from build123d import *

# Parameters (mm, degrees)
CIRPATTERN1_COUNT        = 8
LPATTERN1_START          = -24.818843944
LPATTERN1_OUTLINE_R      = 41.275
LPATTERN1_OUTLINE_R_2    = 38.453474767
LPATTERN1_DEPTH          = 5.187687888
LPATTERN1_START_2        = -12.118843944
LPATTERN1_2_OUTLINE_R    = 41.275
LPATTERN1_2_OUTLINE_R_2  = 38.453474767
LPATTERN1_2_DEPTH        = 5.187687888
Q_0_332_DIAMETER_HOLE1_D = 8.4328


# Read off the part's stored shape, not the designer's step: LPattern1
with BuildPart() as part:
    # Sketch1 → Revolve1 (revolve)
    with BuildSketch(Plane.XY, mode=Mode.PRIVATE) as revolve1_sk:
        Polygon((-41.275, -40.64), (-41.275, 0), (-34.925, 0), (-34.925, -25.4), (-13.91158, -25.4), (-13.91158, -74.93), (-8.90651, -74.93), (-8.90651, -88.392), (-19.05, -88.392), (-19.05, -40.64), align=None)
    revolve(revolve1_sk.sketch.rotate(Axis((0, 0, 0), (0, 1, 0)), 270), axis=Axis((0, 0, 0), (0, 1, 0)))

    # Sketch8 → 1/4-20 Tapped Hole1 (revolve, cut)
    with BuildSketch(Plane(origin=(38.133127704, -34.29, -15.795258671), x_dir=(-0.38268343236509045, 0, -0.9238795325112865), z_dir=(0, 1, 0))):
        Polygon((0, 0), (0, 20.583816902), (2.5527, 19.05), (2.5527, 0), align=None)
    f_1_4_20_tapped_hole1 = revolve(axis=Axis((43.999762736, -34.29, -18.225298466), (-0.9238795325112865, 0, 0.38268343236509045)), mode=Mode.SUBTRACT)

    # CirPattern1: 1/4-20 Tapped Hole1 ×8 about axis
    cirpattern1_axis = Axis((0, -118.183018713, 0), (0, 1, 0))
    for i in range(1, CIRPATTERN1_COUNT):
        add(f_1_4_20_tapped_hole1.rotate(cirpattern1_axis, i * 360 / CIRPATTERN1_COUNT), mode=Mode.SUBTRACT)

    # LPattern1 outline → LPattern1 (cut)
    with BuildSketch(Plane(origin=(0, 0, 0), x_dir=(1, 0, 0), z_dir=(0, 1, 0)).offset(LPATTERN1_START)):
        Circle(LPATTERN1_OUTLINE_R)
        Circle(LPATTERN1_OUTLINE_R_2, mode=Mode.SUBTRACT)
    extrude(amount=LPATTERN1_DEPTH, mode=Mode.SUBTRACT)

    # LPattern1 2 outline → LPattern1 2 (cut)
    with BuildSketch(Plane(origin=(0, 0, 0), x_dir=(1, 0, 0), z_dir=(0, 1, 0)).offset(LPATTERN1_START_2)):
        Circle(LPATTERN1_2_OUTLINE_R)
        Circle(LPATTERN1_2_OUTLINE_R_2, mode=Mode.SUBTRACT)
    extrude(amount=LPATTERN1_2_DEPTH, mode=Mode.SUBTRACT)

    # Q (0.332) Diameter Hole1 (through all)
    with Locations(Plane(origin=(0, -40.64, 0), x_dir=(-1, 0, 0), z_dir=(0, -1, 0))):
        with Locations((0, 29.21)):
            Hole(Q_0_332_DIAMETER_HOLE1_D / 2)


solid = part.part
Geometry check sheet. Reference: the model listing, model coordinates, mm. A direction names the side the tool comes from. Coordinates: 2 decimals unless noted, no trailing zeros. Order: outer loops, then holes, each group sorted by start corner. A loop starts at its lowest first (then second) coordinate and runs counter-clockwise, first axis right, second up. Notation, with made-up numbers: M 58.25,9 L 90.25,9 A29 cw 90.25,33 Z; hole C 59.25,52 d7. An arc over 180 degrees is marked long. Use CSV: the item, a comma, the result in double quotes.
Item 1: Cross-section at C-C on y = -77.5. Record the cut outline in (x, z), then the cut area to 3 significant figures.
Returned:
outline,"C 0,0 d38.1; hole C 0,0 d17.81"
area,"891 mm2"
Item 2: Thickness scan on line 1 along X through (y, z) = (-78, 0); line 2 along X through (y, z) = (-8, 0) (3 decimals); line 3 along Y through (x, z) = (37.5, 12). Record the ranges inside material, lowest first.
Returned:
line 1,"x = -19.05 to -8.91, 8.91 to 19.05"
line 2,"x = -38.453 to -34.925, 34.925 to 38.453"
line 3,"y = -40.64 to -24.82, -19.63 to -12.12, -6.93 to 0"
Item 3: Gauge pin test, flat ends, axial feed: pin 1 Ø22.5 at (x, z) = (-1.5, -4.5) entering from +Y; pin 2 Ø6 at (y, z) = (-29, -25.5) entering from +X; pin 3 Ø7.5 at (x, z) = (0, -29.21) entering from -Y; pin 4 Ø1.5 at (x, y) = (16.5, -28.5) entering from +Z. Record the tip position at first contact, or that the pin passes through.
Returned:
pin 1,"stops at y = -25.4"
pin 2,"stops at x = 34.6"
pin 3,"passes through"
pin 4,"stops at z = 38.15"
Item 4: Tool access check on faces 1 (the flat face through (9, -40.64, 18)), 2 (the cylindrical face through (-12.4, -3.42, -39.37)), 3 (the flat face through (9.1, -74.93, 0.2)), 4 (the conical face through (19.34, -34.73, 8.07)). Record the directions out of +Z, -Z, +X, -X, +Y, -Y that give a thin tool (end or side, any length) a straight path to the whole face; none if there is none.
Returned:
face 1,"-Y"
face 2,"+Y, -Y"
face 3,"+Y"
face 4,"none"
Item 5: Cross-section at D-D on y = -57. Record the cut outline in (x, z).
Returned:
outline,"C 0,0 d38.1; hole C 0,0 d27.82"
Item 6: Mould release check, pull along X, two halves, no side actions. Record for faces 5 (the cylindrical face through (2.267, -32.913, -32.765)), 6 (the cylindrical face through (11.59, -64.18, 15.12)), 7 (the flat face through (4, -88.392, 8.2)): pulls with the +X half, pulls with the -X half, needs draft (parallel to the pull), parting line crosses it, or undercut.
Returned:
face 5,"undercut"
face 6,"parting line crosses it"
face 7,"needs draft"
Item 7: Cross-section at A-A on x = 0. Give the number of separate pieces and of enclosed holes in the cut face, then the cut area to 3 significant figures.
Returned:
separate pieces,"3"
enclosed holes,"0"
area,"1,600 mm2"
